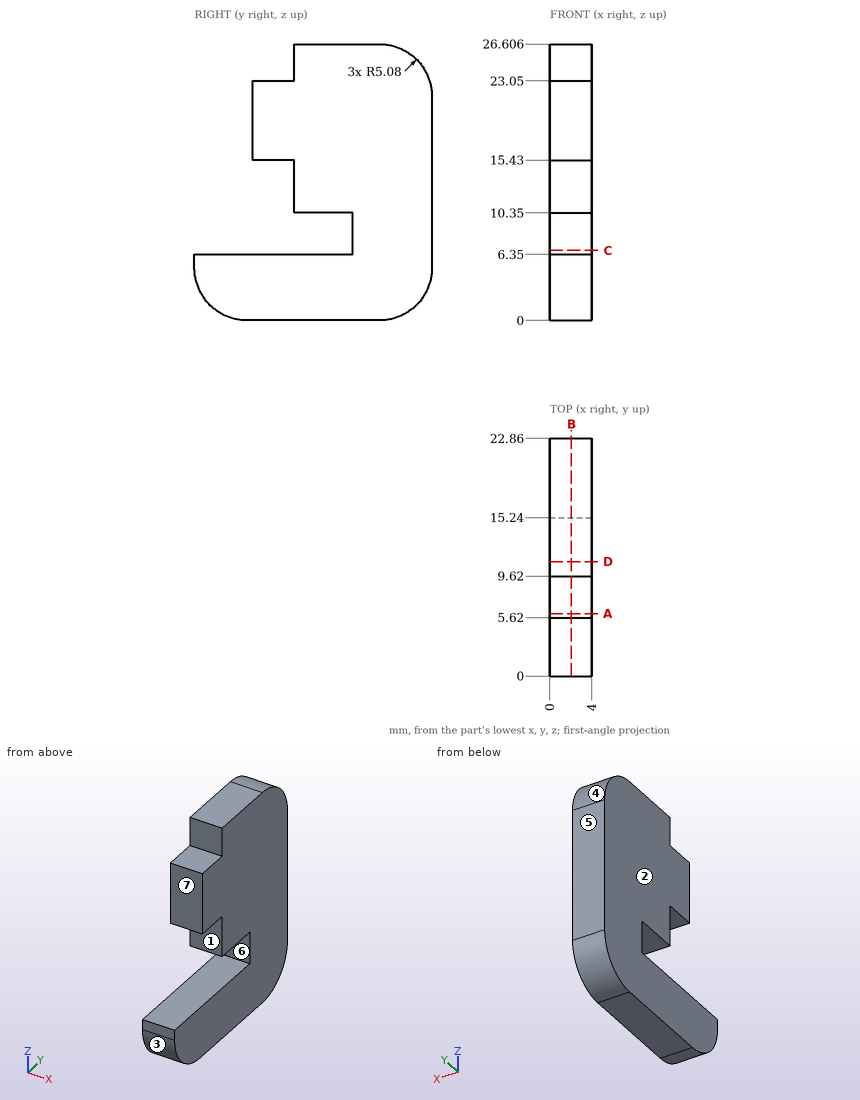
Here's the drawing with two shaded views (mm, measured from the low corner). I have some questions. A direction names the side the tool comes from. Coordinates: 2 decimals unless noted, no trailing zeros. Order: outer loops, then holes, each group sorted by start corner. A loop starts at its lowest first (then second) coordinate and runs counter-clockwise, first axis right, second up. Notation, with made-up numbers: M 66,-38.75 L 91,-38.75 A22 cw 91,-23.75 Z; hole C -33.5,76 d1. An arc over 180 degrees is marked long. Write item = value, one per line.
(1) Suppose I cut it at A-A on y = 6. Please give me the cut outline in (x, z).
Results are:
outline = M 0,0 L 4,0 L 4,6.35 L 0,6.35 Z; M 0,15.43 L 4,15.43 L 4,23.05 L 0,23.05 Z
(2) For pin 1 Ø1 at (y, z) = (11.5, 16) entering from -X; pin 2 Ø1.5 at (x, y) = (3, 19.5) entering from -Z; pin 3 Ø1.2 at (x, y) = (3, 4) entering from +Z; pin 4 Ø1.2 at (x, z) = (2, 8) entering from -Y, each with a flat end and sliding along its axis, tell me the tip position at first contact or that it passes through.
Results are:
pin_1 = 0
pin_2 = 0.09
pin_3 = 6.35
pin_4 = 15.24
(3) For the marked faces 5, 6 and 7, which set-ups out of +Z, -Z, +X, -X, +Y, -Y let a thin tool reach every point of the face, with its end or its side?
Results are:
face_5 = +Z, -Z, +X, -X, +Y
face_6 = +X, -X, -Y
face_7 = +Z, +X, -X, -Y
(4) If we mould it in two halves opening along Z, with no side actions, what happens to the marked faces 1, 2, 3 and 4? For each: pulls with the +Z half, pulls with the -Z half, needs draft (parallel to the pull), parting line crosses it, or undercut.
Results are:
face_1 = undercut
face_2 = needs draft
face_3 = pulls with the -Z half
face_4 = pulls with the +Z half
(5) I need wall thicknesses on line 1 along Z through (x, y) = (2.5, 14); line 2 along Z through (x, y) = (1.3, 6.5); line 3 along Y through (x, z) = (3, 17.75). Which ranges of each line are inside material? Lowest first, please. Write a range as [from, to].
Results are:
line_1 = [0, 6.35], [10.35, 26.61]
line_2 = [0, 6.35], [15.43, 23.05]
line_3 = [5.62, 22.86]
(6) Suppose I cut it at C-C on z = 6.75. Please give me the cut outline in (x, y).
Results are:
outline = M 0,15.24 L 4,15.24 L 4,22.86 L 0,22.86 Z
(7) Suppose I cut it at D-D on y = 11. Please give me the cut outline in (x, z).
Results are:
outline = M 0,0 L 4,0 L 4,6.35 L 0,6.35 Z; M 0,10.35 L 4,10.35 L 4,26.61 L 0,26.61 Z
(8) Suppose I cut it at B-B on x = 2.05. Please give me the cut outline in (y, z).
Results are:
outline = M 0,5.08 A5.08 ccw 5.08,0 L 17.78,0 A5.08 ccw 22.86,5.08 L 22.86,21.53 A5.08 ccw 17.78,26.61 L 9.62,26.61 L 9.62,23.05 L 5.62,23.05 L 5.62,15.43 L 9.62,15.43 L 9.62,10.35 L 15.24,10.35 L 15.24,6.35 L 0,6.35 Z
